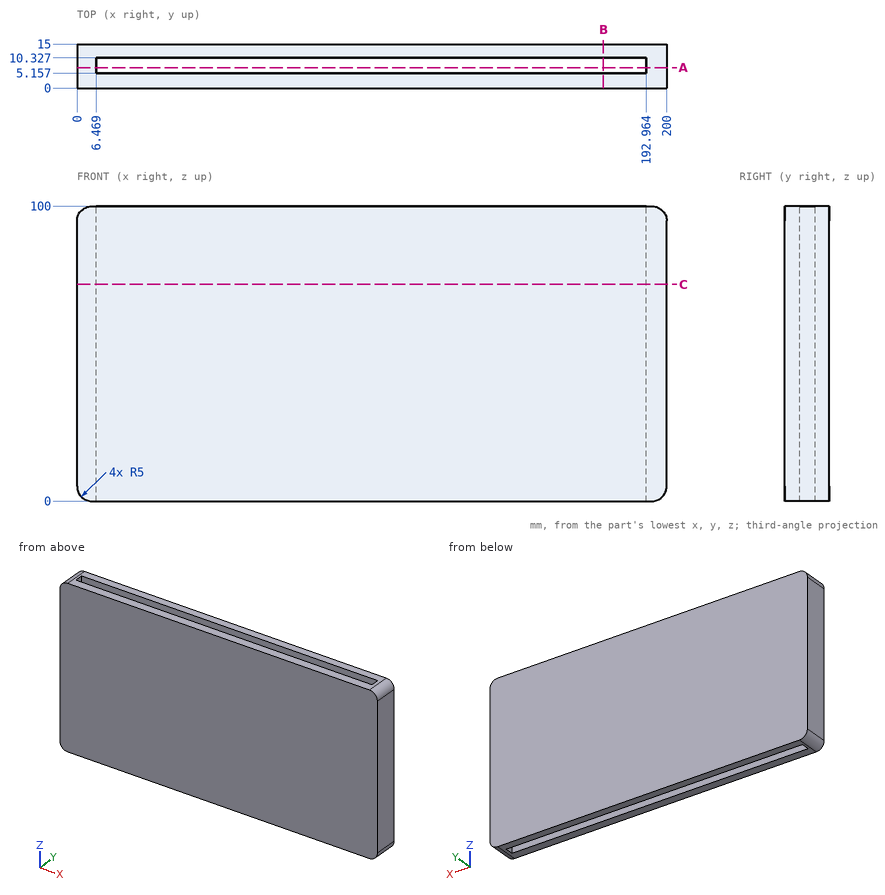
Print and shaded views of the part. All mm, measured from the part's lowest x, y and z. Coordinates: 2 decimals unless noted, no trailing zeros. Order: outer loops, then holes, each group sorted by start corner. A loop starts at its lowest first (then second) coordinate and runs counter-clockwise, first axis right, second up.
Item 1: Saw through at A-A on y = 7. List the corners of the cut face in (x, z).
Filled in:
outline: (0, 5) arc R5 ccw to (5, 0) - (6.47, 0) - (6.47, 100) - (5, 100) arc R5 ccw to (0, 95) - close; (192.96, 0) - (195, 0) arc R5 ccw to (200, 5) - (200, 95) arc R5 ccw to (195, 100) - (192.96, 100) - close
Item 2: Saw through at B-B on x = 178.5. List the corners of the cut face in (y, z).
Filled in:
outline: (0, 0) - (5.16, 0) - (5.16, 100) - (0, 100) - close; (10.33, 0) - (15, 0) - (15, 100) - (10.33, 100) - close
Item 3: Saw through at C-C on z = 73.5. List the corners of the cut face in (x, y), then the cut area to 3 significant figures.
Filled in:
outline: (0, 0) - (200, 0) - (200, 15) - (0, 15) - close; hole (6.47, 5.16) - (192.96, 5.16) - (192.96, 10.33) - (6.47, 10.33) - close
area: 2,040 mm2
Item 4: Drill centre lines: L1, parallel to X at y = 7.5, z = 63.5; L2, parallel to Y at x = 51, z = 54; L3, parallel to X at y = 3.5, z = 95.5 (1 decimal). Where is each one in solid material? Low to high.
Filled in:
L1: x = 0 to 6.47, 192.96 to 200
L2: y = 0 to 5.16, 10.33 to 15
L3: x = 0 to 200
